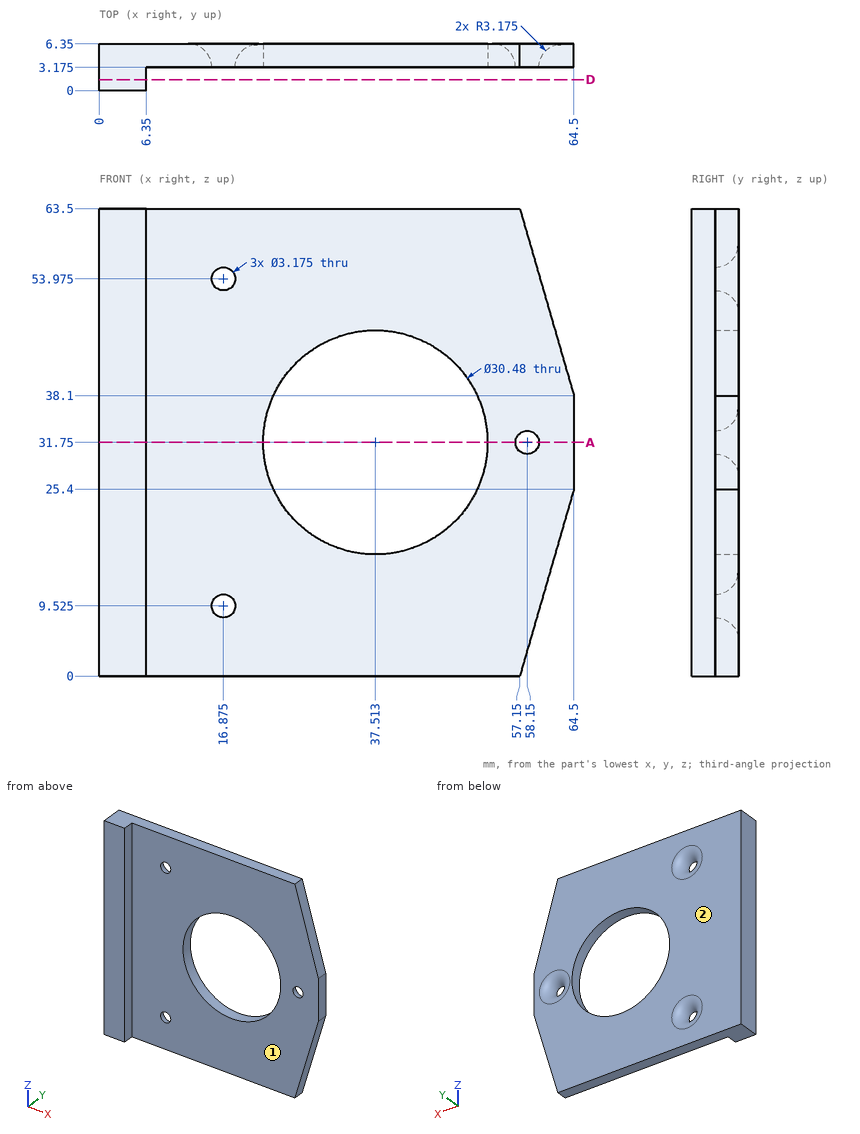
Here's the drawing with two shaded views (mm, measured from the low corner). I have some questions. A direction names the side the tool comes from. Give positions to 0.01 mm unless a question says otherwise; leave off trailing zeros. Order: outer loops, then holes, each group sorted by start corner. A loop starts at its lowest first (then second) coordinate and runs counter-clockwise, first axis right, second up. Notation, with made-up numbers: M -37.75,89 L 17.25,89 A19 cw 17.25,96 Z; hole C -4.5,2.25 d1. An arc over 180 degrees is marked long. One line per item, written item: value.
1) I want a section at D-D, the plane y = 1.5. List the corners of the cut face in (x, z) for me.
Answer sheet:
outline: M 0,0 L 6.35,0 L 6.35,63.5 L 0,63.5 Z
2) I want a section at A-A, the plane z = 31.75. Count the separate pieces of the cut face and the enclosed holes in it, plus the area to 3 significant figures.
Answer sheet:
separate pieces: 3
enclosed holes: 0
area: 114 mm^2
3) Please list where these lines run through material, in increasing order: line 1 along X through (y, z) = (5, 55); line 2 along X through (y, z) = (1.5, 9); line 3 along Z through (x, y) = (18, 3.5).
Answer sheet:
line 1: x = 0 to 14.97, 18.78 to 59.61
line 2: x = 0 to 6.35
line 3: z = 0 to 8.38, 10.67 to 52.83, 55.12 to 63.5
4) For P1, Ø2.5, axis at x = 58.15, z = 31.75, coming from the +Y side; P2, Ø2, axis at y = 1, z = 32.5, coming from the +X side; P3, Ø3, axis at y = 3, z = 20, coming from the +X side, each with a flat end and sliding along its axis, tell me the tip position at first contact or that it passes through.
Answer sheet:
P1: passes through
P2: stops at x = 6.35
P3: stops at x = 63.37
5) On a 3-axis mill with a long thin cutter (end or side, diameter ignored), from which of +Z, -Z, +X, -X, +Y, -Y can I reach the whole of each face in a straight line? I mean the marked faces 1 and 2. Say none if no direction works.
Answer sheet:
face 1: +Z, -Z, +X, -Y
face 2: +Z, -Z, +X, -X, +Y
